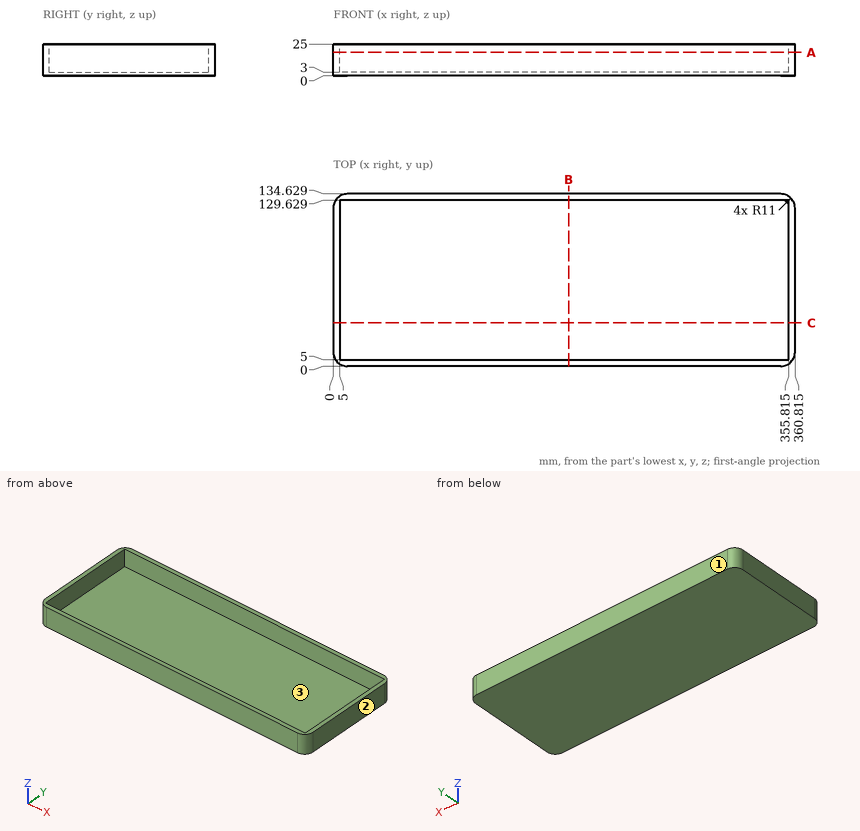
Job drawing, mm, ordinate dimensions from the low corner. One solid piece. Coordinates: 2 decimals unless noted, no trailing zeros. Order: outer loops, then holes, each group sorted by start corner. A loop starts at its lowest first (then second) coordinate and runs counter-clockwise, first axis right, second up. Notation, with made-up numbers: (-37.75, 56) -> (4.25, 56) arc R33 cw to (4.25, 91) -> close; hole circle Ø1 at (-8.75, 67). An arc over 180 degrees is marked (long way). Answer in a Markdown table with one row per item. Add a question column.
Q1. Band-saw the part on B-B, the plane x = 184. List the corners of the cut face in (y, z).
Q2. Wall check: line 1 along Y through (x, z) = (327.5, 9.75); line 2 along X through (y, z) = (19, 8.75) (3 decimals); line 3 along Z through (x, y) = (237.5, 97.5). Give the ranges that are in metal, low to high. Write a range as [from, to].
Q3. Mould opens along X. For the marked faces 1, 2 and 3 say: +X half, -X half, draft (parallel to the pull), parting line (faces both ways), or undercut.
Q4. Drop a flat-ended pin along its axis: pin 1 (6 mm diameter, centred on x = 189.5, y = 93, fed in from +Z). Give the stop position or say it passes through.
Q5. Band-saw the part on C-C, the plane y = 34. List the corners of the cut face in (x, z) (3 decimals).
Q6. Band-saw the part on A-A, the plane z = 18.5. List the corners of the cut face in (x, y) (3 decimals).
Answers follow:
| question | item | result |
|---|---|---|
| 1 | outline | (0, 0) -> (134.63, 0) -> (134.63, 25) -> (129.63, 25) -> (129.63, 3) -> (5, 3) -> (5, 25) -> (0, 25) -> close |
| 2 | line 1 | [0, 5], [129.63, 134.63] |
| 2 | line 2 | [0, 5], [355.815, 360.815] |
| 2 | line 3 | [0, 3] |
| 3 | face 1 | draft |
| 3 | face 2 | +X half |
| 3 | face 3 | undercut |
| 4 | pin 1 | z = 3 |
| 5 | outline | (0, 0) -> (360.815, 0) -> (360.815, 25) -> (355.815, 25) -> (355.815, 3) -> (5, 3) -> (5, 25) -> (0, 25) -> close |
| 6 | outline | (0, 11) arc R11 ccw to (11, 0) -> (349.815, 0) arc R11 ccw to (360.815, 11) -> (360.815, 123.629) arc R11 ccw to (349.815, 134.629) -> (11, 134.629) arc R11 ccw to (0, 123.629) -> close; hole (5, 5) -> (355.815, 5) -> (355.815, 129.629) -> (5, 129.629) -> close |
